Here's how the part is built. I have some questions about the finished solid (model axes, mm). Face numbers are marked on the shaded views. A direction names the side the tool comes from. Coordinates: 2 decimals unless noted, no trailing zeros. Write each loop counter-clockwise with the first axis right and the second up, starting at its lowest first coordinate (ties: lowest second). Pieces come first, ordered by that corner, then holes. Notation, with made-up numbers: (86.5, -40) -> (103.5, -40) arc R25 cw to (103.5, -20) -> close; hole circle Ø9 at (-25.75, -14.5). An arc over 180 degrees is marked (long way). Put each result on its own line as item: value.
```python
from build123d import *

# Parameters (mm, degrees)
BOSS_EXTRUDE1_DEPTH = 15.875
CUT_EXTRUDE1_REACH  = 150.955
SKETCH2_R           = 3.175
CUT_EXTRUDE2_REACH  = 150.955
SKETCH3_R           = 3.175


with BuildPart() as part:
    # Sketch1 → Boss-Extrude1 (new, symmetric)
    with BuildSketch(Plane(origin=(0, 0, 0), x_dir=(1, 0, 0), z_dir=(0, 1, 0))):
        Polygon((-50.8, 0), (50.8, 0), (63.5, 12.7), (63.5, 76.2), (-63.5, 76.2), (-63.5, 12.7), align=None)
        Polygon((60.325, 73.025), (-60.325, 73.025), (-60.325, 14.015128061), (-49.484871939, 3.175), (49.484871939, 3.175), (60.325, 14.015128061), align=None, mode=Mode.SUBTRACT)
    extrude(amount=BOSS_EXTRUDE1_DEPTH, both=True)

    # Sketch2 → Cut-Extrude1 (cut, up to next)
    with BuildSketch(Plane.ZY.offset(63.5), mode=Mode.PRIVATE) as cut_extrude1_sk1:
        with Locations((-28.575, 0)):
            Circle(SKETCH2_R)
    cut_extrude1_tool1 = extrude(cut_extrude1_sk1.sketch, amount=-CUT_EXTRUDE1_REACH, mode=Mode.PRIVATE) & part.part
    add(cut_extrude1_tool1.solids().sort_by_distance((-63.5, 0, -28.575))[0], mode=Mode.SUBTRACT)

    # Sketch3 → Cut-Extrude2 (cut, up to next)
    with BuildSketch(Plane(origin=(63.5, 0, 0), x_dir=(0, 0, -1), z_dir=(1, 0, 0)), mode=Mode.PRIVATE) as cut_extrude2_sk1:
        with Locations(Location((28.575, 0, 0), (0, 0, 180))):
            Circle(SKETCH3_R)
    cut_extrude2_tool1 = extrude(cut_extrude2_sk1.sketch, amount=-CUT_EXTRUDE2_REACH, mode=Mode.PRIVATE) & part.part
    add(cut_extrude2_tool1.solids().sort_by_distance((63.5, 0, -28.575))[0], mode=Mode.SUBTRACT)


solid = part.part
```
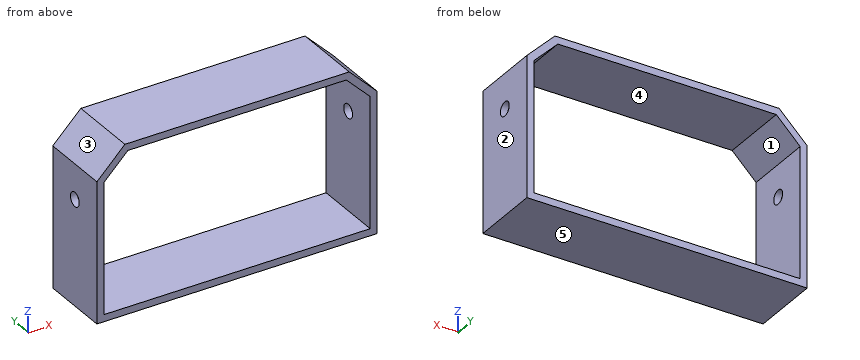
Item 1: Imagine slicing it at B-B on z = -68. Write out the boundary of the cut face in (x, y) (3 decimals), then the cut area to 3 significant figures.
Output:
outline: (-63.5, -15.875) -> (-60.325, -15.875) -> (-60.325, 15.875) -> (-63.5, 15.875) -> close; (60.325, -15.875) -> (63.5, -15.875) -> (63.5, 15.875) -> (60.325, 15.875) -> close
area: 202 mm²
Item 2: Which directions (+Z, -Z, +X, -X, +Y, -Y) give clear straight access to the entire face, cutting with the end or side of a thin tool? Please do the marked faces 1 and 2.
Output:
face 1: +Y, -Y
face 2: +Z, -Z, +X, +Y, -Y
Item 3: If we mould it in two halves opening along Z, with no side actions, what happens to the marked faces 3, 4 and 5? For each: released by +Z, released by -Z, zero draft, split by the parting line, or undercut.
Output:
face 3: released by +Z
face 4: undercut
face 5: released by -Z
Item 4: Please list where these lines run through material, in increasing order: line 1 along Z through (x, y) = (36, 9.5) (3 decimals); line 2 along X through (y, z) = (9.5, -23) (3 decimals); line 3 along X through (y, z) = (1.5, -9.5). Write a range as from..to.
Output:
line 1: z = -76.2..-73.025, -3.175..0
line 2: x = -63.5..-60.325, 60.325..63.5
line 3: x = -60.3..-55.81, 55.81..60.3
Item 5: Imagine slicing it at A-A on x = -36.5. Write out the boundary of the cut face in (y, z) (3 decimals), then the cut area to 3 significant figures.
Output:
outline: (-15.875, -76.2) -> (15.875, -76.2) -> (15.875, -73.025) -> (-15.875, -73.025) -> close; (-15.875, -3.175) -> (15.875, -3.175) -> (15.875, 0) -> (-15.875, 0) -> close
area: 202 mm²
Item 6: Imagine slicing it at C-C on y = 0. Write out the boundary of the cut face in (x, z) (3 decimals), then the cut area to 3 significant figures.
Output:
outline: (-63.5, -76.2) -> (63.5, -76.2) -> (63.5, -31.75) -> (60.325, -31.75) -> (60.325, -73.025) -> (-60.325, -73.025) -> (-60.325, -31.75) -> (-63.5, -31.75) -> close; (-63.5, -25.4) -> (-60.325, -25.4) -> (-60.325, -14.015) -> (-49.485, -3.175) -> (49.485, -3.175) -> (60.325, -14.015) -> (60.325, -25.4) -> (63.5, -25.4) -> (63.5, -12.7) -> (50.8, 0) -> (-50.8, 0) -> (-63.5, -12.7) -> close
area: 1,170 mm²
Item 7: For P1, Ø4, axis at x = 8.5, y = 5, coming from the +Z side, with a flat end and sliding along its axis, tell me the tip position at first contact or that it passes through.
Output:
P1: stops at z = 0
Item 8: Imagine slicing it at D-D on y = 7. Write out the boundary of the cut face in (x, z) (3 decimals).
Output:
outline: (-63.5, -76.2) -> (63.5, -76.2) -> (63.5, -12.7) -> (50.8, 0) -> (-50.8, 0) -> (-63.5, -12.7) -> close; hole (-60.325, -73.025) -> (60.325, -73.025) -> (60.325, -14.015) -> (49.485, -3.175) -> (-49.485, -3.175) -> (-60.325, -14.015) -> close
